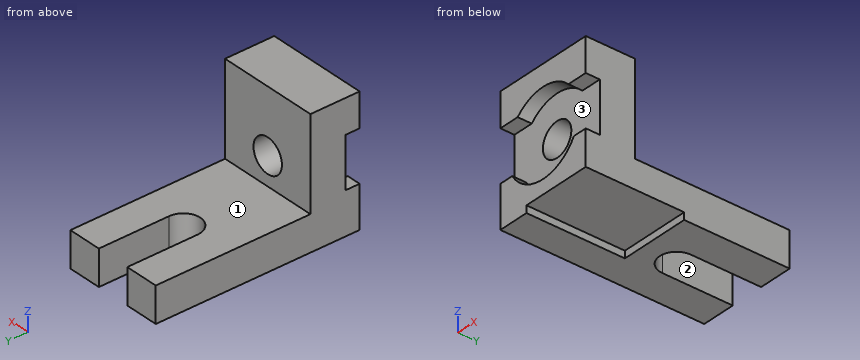
```python
from build123d import *

# Parameters (mm, degrees)
SKETCH_W        = 72
SKETCH_H        = 145
PAD_DEPTH       = 25
SKETCH001_W     = 72
SKETCH001_H     = 35
PAD001_DEPTH    = 65
SKETCH002_W     = 70
SKETCH002_H     = 18.58303
POCKET_DEPTH    = 50
POCKET001_DEPTH = 25.001
SKETCH004_R     = 12
POCKET002_DEPTH = 145.001
SKETCH005_R     = 30
POCKET003_DEPTH = 10
SKETCH006_W     = 22.449348
SKETCH006_H     = 36
POCKET004_DEPTH = 72.001


with BuildPart() as part:
    # Sketch → Pad (new body)
    with BuildSketch(Plane.XY):
        Rectangle(SKETCH_W, SKETCH_H)
    extrude(amount=PAD_DEPTH)

    # Sketch001 → Pad001 (new body)
    with BuildSketch(Plane.XY.offset(25)):
        with Locations((0, -55)):
            Rectangle(SKETCH001_W, SKETCH001_H)
    extrude(amount=PAD001_DEPTH)

    # Sketch002 → Pocket (cut)
    with BuildSketch(Plane.YZ.offset(36)):
        with Locations((-37.5, -4.291515)):
            Rectangle(SKETCH002_W, SKETCH002_H)
    extrude(amount=-POCKET_DEPTH, mode=Mode.SUBTRACT)

    # Sketch003 → Pocket001 (cut, through all)
    with BuildSketch(Plane.XY.offset(25)):
        with BuildLine():
            ThreePointArc((-12, 22.5), (0, 10.5), (12, 22.5))
            Line((12, 22.5), (12, 75.823228))
            ThreePointArc((12, 75.823228), (0, 87.823228), (-12, 75.823228))
            Line((-12, 22.5), (-12, 75.823228))
        make_face()
    extrude(amount=-POCKET001_DEPTH, mode=Mode.SUBTRACT)

    # Sketch004 → Pocket002 (cut, through all)
    with BuildSketch(Plane.XZ.offset(72.5)):
        with Locations((0, 45)):
            Circle(SKETCH004_R)
    extrude(amount=-POCKET002_DEPTH, mode=Mode.SUBTRACT)

    # Sketch005 → Pocket003 (cut)
    with BuildSketch(Plane.XZ.offset(72.5)):
        with Locations((0, 45)):
            Circle(SKETCH005_R)
    extrude(amount=-POCKET003_DEPTH, mode=Mode.SUBTRACT)

    # Sketch006 → Pocket004 (cut, through all)
    with BuildSketch(Plane.YZ.offset(36)):
        with Locations((-73.724674, 48)):
            Rectangle(SKETCH006_W, SKETCH006_H)
    extrude(amount=-POCKET004_DEPTH, mode=Mode.SUBTRACT)


solid = part.part
```
Geometry check sheet. Reference: the model listing, model coordinates, mm. Face numbers are marked on the shaded views. A direction names the side the tool comes from. Round coordinates to 2 decimals unless told otherwise and drop trailing zeros. Loops run counter-clockwise (first coordinate to the right, second up) from the corner with the lowest first, then second, coordinate; pieces in that order, holes last. Notation, with made-up numbers: (84, 76) -> (106, 76) arc R24 cw to (106, 112) -> close; hole circle Ø4 at (81, -38). An arc over 180 degrees is marked (long way). Use a Markdown table: item, result.
(1) Set-up check for the marked faces 1, 2 and 3: record each of +Z, -Z, +X, -X, +Y, -Y from which the full face is reachable in a straight line by a thin tool's end or side.
Calculated:
| item | result |
|---|---|
| face 1 | +Z, +X, -X, +Y |
| face 2 | +Z, -Z, +Y |
| face 3 | -Y |
(2) Sectioned sample at C-C (z = 45). Enter the section's corners in (x, y), then the cut area to 3 significant figures.
Calculated:
| item | result |
|---|---|
| outline | (-36, -62.5) -> (-12, -62.5) -> (-12, -37.5) -> (-36, -37.5) -> close; (12, -62.5) -> (36, -62.5) -> (36, -37.5) -> (12, -37.5) -> close |
| area | 1,200 mm² |
(3) Go/stop test with flat-tipped pins: P1, Ø10, axis at x = 27.5, y = -35, coming from the -Z side; P2, Ø2.5, axis at x = 10.5, z = 2, coming from the -Y side; P3, Ø3, axis at x = 28.5, y = -28.5, coming from the +Z side; P4, Ø6, axis at y = 37, z = 29.5, coming from the +X side. Record where each tip stops, or that it passes through.
Calculated:
| item | result |
|---|---|
| P1 | z = 5 |
| P2 | y = -2.5 |
| P3 | z = 25 |
| P4 | through |
(4) Sectioned sample at B-B (x = 0). Enter the section's corners in (y, z).
Calculated:
| item | result |
|---|---|
| outline | (-72.5, 5) -> (-2.5, 5) -> (-2.5, 0) -> (10.5, 0) -> (10.5, 25) -> (-37.5, 25) -> (-37.5, 33) -> (-62.5, 33) -> (-62.5, 15) -> (-72.5, 15) -> close; (-72.5, 75) -> (-62.5, 75) -> (-62.5, 57) -> (-37.5, 57) -> (-37.5, 90) -> (-72.5, 90) -> close |
(5) Sectioned sample at D-D (y = -56). Enter the section's corners in (x, z), then the cut area to 3 significant figures.
Calculated:
| item | result |
|---|---|
| outline | (-36, 0) -> (-14, 0) -> (-14, 5) -> (36, 5) -> (36, 90) -> (-36, 90) -> close; hole circle Ø24 at (0, 45) |
| area | 5,780 mm² |
(6) Scan lines: probe 1 along Z at (x, y) = (0, -46.5); probe 2 along Y at (x, z) = (31, 82.5); probe 3 along Y at (x, z) = (-14.5, 62.5). Record each from-to range of solid material in increasing order.
Calculated:
| item | result |
|---|---|
| probe 1 | 5 to 33, 57 to 90 |
| probe 2 | -72.5 to -37.5 |
| probe 3 | -62.5 to -37.5 |
(7) Sectioned sample at A-A (y = 38). Enter the section's corners in (x, z), then the cut area to 3 significant figures.
Calculated:
| item | result |
|---|---|
| outline | (-36, 0) -> (-12, 0) -> (-12, 25) -> (-36, 25) -> close; (12, 0) -> (36, 0) -> (36, 25) -> (12, 25) -> close |
| area | 1,200 mm² |
